from build123d import *

# Parameters (mm, degrees)
F0_W     = 50
F0_H     = 39.1
F1_DEPTH = 6
F2_W     = 50
F2_H     = 5.7
F3_DEPTH = 3.1
F4_DEPTH = 12
F5_R     = 2


with BuildPart() as f1:
    # F0 (on Top) → F1 (new body, symmetric)
    with BuildSketch(Plane.XY):
        Rectangle(F0_W, F0_H)
    extrude(amount=F1_DEPTH, both=True)

    # F2 (on face) → F3 (cut)
    with BuildSketch(Plane.XY.offset(6)):
        with Locations((0, 12.35)):
            Rectangle(F2_W, F2_H)
    extrude(amount=-F3_DEPTH, mode=Mode.SUBTRACT)

    # F2 (on face) → F4 (cut, through all)
    with BuildSketch(Plane.XY.offset(6)):
        with BuildLine():
            Line((25, -4.1), (25, 0))
            Line((25, 0), (25, 4.1))
            Line((25, 4.1), (18.1580818318, 4.1))
            ThreePointArc((18.1580818318, 4.1), (6.5, 0), (18.1580818318, -4.1))
            Line((18.1580818318, -4.1), (25, -4.1))
        make_face()
    extrude(amount=-F4_DEPTH, mode=Mode.SUBTRACT)

    # F5
    f5_edges = [f1.edges().sort_by_distance(p)[0] for p in [
        (0, -19.55, 6),
        (0, 15.2, 6),
        (0, 19.55, 6),
    ]]
    fillet(f5_edges, radius=F5_R)


solid = f1.part
Verification items for the finished model (mm, model axes). A direction names the side the tool comes from. Coordinates: 2 decimals unless noted, no trailing zeros. Write each loop counter-clockwise with the first axis right and the second up, starting at its lowest first coordinate (ties: lowest second). Pieces come first, ordered by that corner, then holes. Notation, with made-up numbers: M 66.25,-1 L 103.25,-1 A24 cw 103.25,30 Z; hole C 30,-3 d10. An arc over 180 degrees is marked long. One line per question, with ' | ' between items.
1) Release check for a two-part mould opening along Y. For faces 4 (the face through (0, -19.55, -1)), 5 (the face through (0, 0, -6)), 6 (the face through (0, 9.5, 4)) record: +Y half, -Y half, draft (parallel to the pull), parting line (faces both ways), or undercut.
Solutions:
face 4: -Y half | face 5: draft | face 6: undercut
2) Sectioned sample at A-A on x = 13.05. Record the cut outline in (y, z).
Solutions:
outline: M -19.55,-6 L -6.55,-6 L -6.55,6 L -17.55,6 A2 ccw -19.55,4 Z; M 6.55,-6 L 19.55,-6 L 19.55,4 A2 ccw 17.55,6 L 17.2,6 A2 ccw 15.2,4 L 15.2,2.9 L 9.5,2.9 L 9.5,6 L 6.55,6 Z
3) Material ranges on L1, parallel to Y at x = 13.05, z = 3.25; L2, parallel to Y at x = 13.05, z = 0; L3, parallel to Y at x = -20.5, z = 3, recorded low to high.
Solutions:
L1: -19.55 to -6.55, 6.55 to 9.5, 15.2 to 19.55 | L2: -19.55 to -6.55, 6.55 to 19.55 | L3: -19.55 to 9.5, 15.2 to 19.55
4) Sectioned sample at D-D on z = -5.25. Record the cut outline in (x, y).
Solutions:
outline: M -25,-19.55 L 25,-19.55 L 25,-4.1 L 18.16,-4.1 A6.55 cw long 18.16,4.1 L 25,4.1 L 25,19.55 L -25,19.55 Z
5) Access from +Z, -Z, +X, -X, +Y, -Y to the whole of each face (thin tool, end or side, straight path). Record for faces 1 (the face through (22, 4.1, 0)), 2 (the face through (-0.3, 15.2, 3.5)), 3 (the face through (0.35, 18.95, 5.43)).
Solutions:
face 1: +Z, -Z, +X | face 2: +Z, +X, -X | face 3: +Z, +X, -X, +Y
6) Sectioned sample at C-C on y = -6. Record the cut outline in (x, z).
Solutions:
outline: M -25,-6 L 10.42,-6 L 10.42,6 L -25,6 Z; M 15.68,-6 L 25,-6 L 25,6 L 15.68,6 Z
7) Sectioned sample at B-B on x = 4.5. Record the cut outline in (y, z), then the cut area to 3 significant figures.
Solutions:
outline: M -19.55,-6 L 19.55,-6 L 19.55,4 A2 ccw 17.55,6 L 17.2,6 A2 ccw 15.2,4 L 15.2,2.9 L 9.5,2.9 L 9.5,6 L -17.55,6 A2 ccw -19.55,4 Z | area: 449 mm^2
